Model file for the job. Use its own axes, mm. Face numbers are marked on the shaded views. Give positions to 0.01 mm unless a question says otherwise; leave off trailing zeros. Order: outer loops, then holes, each group sorted by start corner. A loop starts at its lowest first (then second) coordinate and runs counter-clockwise, first axis right, second up. Notation, with made-up numbers: (71, 45) -> (102, 45) arc R25 cw to (102, 71) -> close; hole circle Ø6 at (70, 41.5). An arc over 180 degrees is marked (long way). Use CSV: the item, a comma, the result in double quotes. Start each with the question number.
1. Pull direction Y, two halves, no side cores. Call the marked faces 1 and 2: released by +Y, released by -Y, zero draft, split by the parting line, or undercut.
2. Cut at D-D on z = 6. Give the number of separate pieces and of enclosed holes in the cut face, then the cut area to 3 significant figures.
3. Drop flat-ended pins along their axis: pin 1 (2.5 mm diameter, centred on x = 56, y = 45, fed in from -Z); pin 2 (1.7 mm diameter, centred on x = -44.5, y = -43, fed in from +Z); pin 3 (3 mm diameter, centred on x = -34, y = -44.5, fed in from -Z). Give the stop position or say it passes through.
4. Wall check: line 1 (Y direction, x = -44, z = 2.9); line 2 (Y direction, x = 44, z = 2.65); line 3 (Y direction, x = -16, z = 4). Give the ranges that are in metal, low to high. Write a range as from..to.
5. Cut at B-B on y = 2.5. List the corners of the cut face in (x, z), then the cut area to 3 significant figures.
6. Cut at C-C on x = 44. List the corners of the cut face in (y, z), then the cut area to 3 significant figures.
7. Cut at A-A on x = 19. List the corners of the cut face in (y, z), then the cut area to 3 significant figures.
```python
from build123d import *

# Parameters (mm, degrees)
SKICA1_W                 = 112
SKICA1_H                 = 100
SKICA1_R                 = 1.6
SKICA1_W_2               = 92
SKICA1_H_2               = 80
P_IDAT_VYSUNUT_M1_DEPTH  = 8
SKICA2_R                 = 2.9
ODEBRAT_VYSUNUT_M1_DEPTH = 4
SKICA3_R                 = 1.6
P_IDAT_VYSUNUT_M2_DEPTH  = 4
ZKOSEN_1_SIZE            = 0.5
ZAOBLIT1_R               = 5
SKICA4_R                 = 4
SKICA4_R_2               = 1.6
P_IDAT_VYSUNUT_M3_DEPTH  = 3


with BuildPart() as part:
    # Skica1 → Přidat vysunutím1 (new body)
    with BuildSketch(Plane.XY):
        with Locations((6, 0)):
            Rectangle(SKICA1_W, SKICA1_H)
        with Locations((-44, 44)):
            Circle(SKICA1_R, mode=Mode.SUBTRACT)
        with Locations((44, 44)):
            Circle(SKICA1_R, mode=Mode.SUBTRACT)
        with Locations((-44, -44)):
            Circle(SKICA1_R, mode=Mode.SUBTRACT)
        with Locations((44, -44)):
            Circle(SKICA1_R, mode=Mode.SUBTRACT)
        Polygon((-34, 41.766838493), (-31.2, 43.383419246), (-31.2, 46.616580754), (-34, 48.233161507), (-36.8, 46.616580754), (-36.8, 43.383419246), align=None, mode=Mode.SUBTRACT)
        Polygon((56, 41.766838493), (58.8, 43.383419246), (58.8, 46.616580754), (56, 48.233161507), (53.2, 46.616580754), (53.2, 43.383419246), align=None, mode=Mode.SUBTRACT)
        Polygon((53.2, -43.383419246), (56, -41.766838493), (58.8, -43.383419246), (58.8, -46.616580754), (56, -48.233161507), (53.2, -46.616580754), align=None, mode=Mode.SUBTRACT)
        Polygon((-36.8, -43.383419246), (-34, -41.766838493), (-31.2, -43.383419246), (-31.2, -46.616580754), (-34, -48.233161507), (-36.8, -46.616580754), align=None, mode=Mode.SUBTRACT)
        with Locations((6, 0)):
            Rectangle(SKICA1_W_2, SKICA1_H_2, mode=Mode.SUBTRACT)
    extrude(amount=P_IDAT_VYSUNUT_M1_DEPTH)

    # Skica2 → Odebrat vysunutím1 (cut)
    with BuildSketch(Plane.XY.offset(8)):
        with Locations((-44, 44)):
            Circle(SKICA2_R)
        with Locations((44, 44)):
            Circle(SKICA2_R)
        with Locations((44, -44)):
            Circle(SKICA2_R)
        with Locations((-44, -44)):
            Circle(SKICA2_R)
    extrude(amount=-ODEBRAT_VYSUNUT_M1_DEPTH, mode=Mode.SUBTRACT)

    # Skica3 → Přidat vysunutím2 (add)
    with BuildSketch(Plane.XY.offset(8)):
        Polygon((-31.2, -46.616580754), (-31.2, -43.383419246), (-34, -41.766838493), (-36.8, -43.383419246), (-36.8, -46.616580754), (-34, -48.233161507), align=None)
        with Locations((-34, -45)):
            Circle(SKICA3_R, mode=Mode.SUBTRACT)
        Polygon((58.8, -46.616580754), (58.8, -43.383419246), (56, -41.766838493), (53.2, -43.383419246), (53.2, -46.616580754), (56, -48.233161507), align=None)
        with Locations((56, -45)):
            Circle(SKICA3_R, mode=Mode.SUBTRACT)
        Polygon((53.2, 46.616580754), (53.2, 43.383419246), (56, 41.766838493), (58.8, 43.383419246), (58.8, 46.616580754), (56, 48.233161507), align=None)
        with Locations((56, 45)):
            Circle(SKICA3_R, mode=Mode.SUBTRACT)
        Polygon((-34, 48.233161507), (-36.8, 46.616580754), (-36.8, 43.383419246), (-34, 41.766838493), (-31.2, 43.383419246), (-31.2, 46.616580754), align=None)
        with Locations((-34, 45)):
            Circle(SKICA3_R, mode=Mode.SUBTRACT)
    extrude(amount=-P_IDAT_VYSUNUT_M2_DEPTH)

    # Zkosení1
    zkosen_1_edges = [part.edges().sort_by_distance(p)[0] for p in [
        (-46.9, -44, 8),
        (41.1, -44, 8),
        (41.1, 44, 8),
        (-46.9, 44, 8),
    ]]
    chamfer(zkosen_1_edges, length=ZKOSEN_1_SIZE)

    # Zaoblit1
    zaoblit1_edges = [part.edges().sort_by_distance(p)[0] for p in [
        (-40, 40, 4),
        (-40, -40, 4),
        (52, -40, 4),
        (52, 40, 4),
        (-50, 50, 4),
        (62, 50, 4),
        (62, -50, 4),
        (-50, -50, 4),
    ]]
    fillet(zaoblit1_edges, radius=ZAOBLIT1_R)

    # Skica4 → Přidat vysunutím3 (add)
    with BuildSketch(Plane.XY.offset(8)):
        with Locations((-34, 45)):
            Circle(SKICA4_R)
        with Locations((-34, 45)):
            Circle(SKICA4_R_2, mode=Mode.SUBTRACT)
        with Locations((56, 45)):
            Circle(SKICA4_R)
        with Locations((56, 45)):
            Circle(SKICA4_R_2, mode=Mode.SUBTRACT)
        with Locations((56, -45)):
            Circle(SKICA4_R)
        with Locations((56, -45)):
            Circle(SKICA4_R_2, mode=Mode.SUBTRACT)
        with Locations((-34, -45)):
            Circle(SKICA4_R)
        with Locations((-34, -45)):
            Circle(SKICA4_R_2, mode=Mode.SUBTRACT)
    extrude(amount=P_IDAT_VYSUNUT_M3_DEPTH)


solid = part.part
```
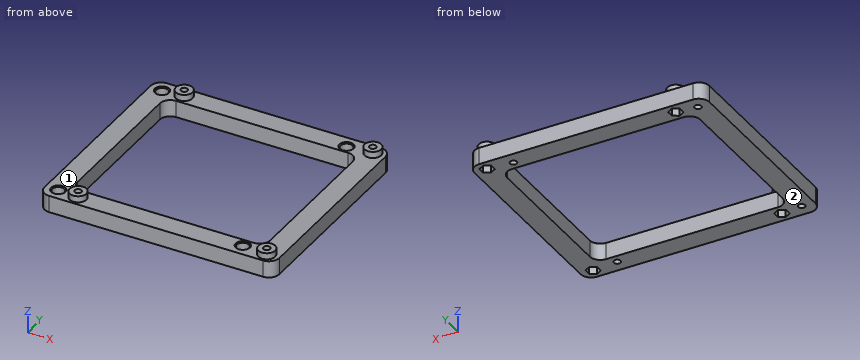
Verdict:
1,face 1,"undercut"
1,face 2,"zero draft"
2,separate pieces,"1"
2,enclosed holes,"9"
2,area,"3,700 mm^2"
3,pin 1,"through"
3,pin 2,"z = 4"
3,pin 3,"z = 4"
4,line 1,"-50..-45.6, -42.4..42.4, 45.6..50"
4,line 2,"-50..-45.6, -42.4..-40, 40..42.4, 45.6..50"
4,line 3,"-50..-40, 40..50"
5,outline,"(-50, 0) -> (-40, 0) -> (-40, 8) -> (-50, 8) -> close; (52, 0) -> (62, 0) -> (62, 8) -> (52, 8) -> close"
5,area,"160 mm^2"
6,outline,"(-50, 0) -> (-45.6, 0) -> (-45.6, 4) -> (-46.9, 4) -> (-46.9, 7.5) -> (-47.4, 8) -> (-50, 8) -> close; (-42.4, 0) -> (-40, 0) -> (-40, 8) -> (-40.6, 8) -> (-41.1, 7.5) -> (-41.1, 4) -> (-42.4, 4) -> close; (40, 0) -> (42.4, 0) -> (42.4, 4) -> (41.1, 4) -> (41.1, 7.5) -> (40.6, 8) -> (40, 8) -> close; (45.6, 0) -> (50, 0) -> (50, 8) -> (47.4, 8) -> (46.9, 7.5) -> (46.9, 4) -> (45.6, 4) -> close"
6,area,"87.5 mm^2"
7,outline,"(-50, 0) -> (-40, 0) -> (-40, 8) -> (-50, 8) -> close; (40, 0) -> (50, 0) -> (50, 8) -> (40, 8) -> close"
7,area,"160 mm^2"
